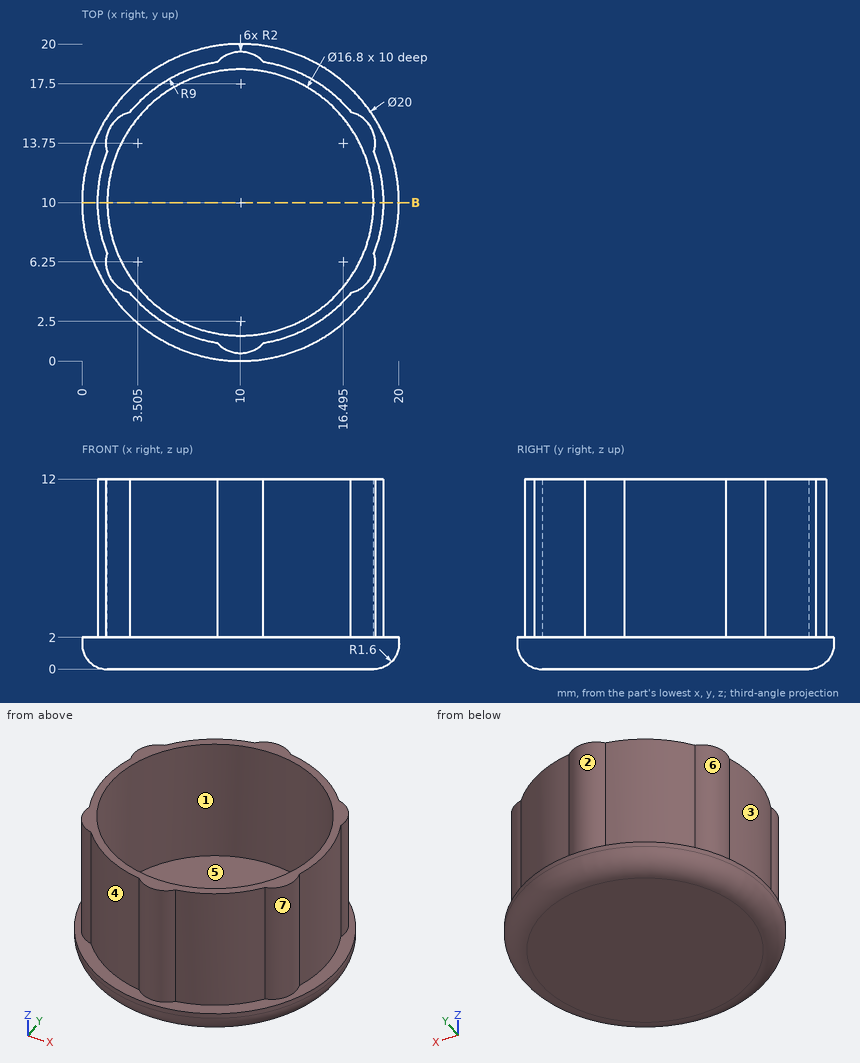
Drawing for the job (mm, zero at the part's lowest x, y, z). A direction names the side the tool comes from. Round coordinates to 2 decimals unless told otherwise and drop trailing zeros. Write each loop counter-clockwise with the first axis right and the second up, starting at its lowest first coordinate (ties: lowest second). Pieces come first, ordered by that corner, then holes. Notation, with made-up numbers: M 88.25,-13 L 103.25,-13 A11 cw 103.25,-2 Z; hole C 11,23.25 d9. An arc over 180 degrees is marked long. Answer in a Markdown table with one row per item.
1. Flat gauge pins, fed straight in: P1, Ø12, axis at x = 4.5, y = 15.5, coming from the -Z side; P2, Ø6, axis at x = 16, z = 10.5, coming from the +Y side (1 decimal); P3, Ø6, axis at x = 3, z = 2.5, coming from the +Y side; P4, Ø4, axis at x = 14, y = 10.5, coming from the +Z side. Where does each tip first touch, or does it go through?
Geometry check:
| item | result |
|---|---|
| P1 | z = 0 |
| P2 | y = 18.5 |
| P3 | y = 19.15 |
| P4 | z = 2 |
2. Saw through at B-B (y = 10). List the corners of the cut face in (x, z), and give its area (3 significant figures).
Geometry check:
| item | result |
|---|---|
| outline | M 0,1.6 A1.6 ccw 1.6,0 L 18.4,0 A1.6 ccw 20,1.6 L 20,2 L 19,2 L 19,12 L 18.4,12 L 18.4,2 L 1.6,2 L 1.6,12 L 1,12 L 1,2 L 0,2 Z |
| area | 50.9 mm2 |
3. Mould opens along X. For the marked faces 1, 2 and 3 say: +X half, -X half, draft (parallel to the pull), parting line (faces both ways), or undercut.
Geometry check:
| item | result |
|---|---|
| face 1 | undercut |
| face 2 | parting line |
| face 3 | -X half |
4. Probe L1, parallel to Z at x = 10.25, y = 9; L2, parallel to X at y = 7.75, z = 10.25; L3, parallel to Y at x = 17.5, z = 9.5. List the from-to ranges inside material, lowest first. Write a range as [from, to].
Geometry check:
| item | result |
|---|---|
| L1 | [0, 2] |
| L2 | [1.29, 1.91], [18.09, 18.71] |
| L3 | [4.52, 6.22], [13.78, 15.48] |
5. Which spindle directions (+Z, -Z, +X, -X, +Y, -Y) get a long thin tool onto all of the face, cutting with end or side? Do the marked faces 4, 5, 6 and 7. Say none if no direction does.
Geometry check:
| item | result |
|---|---|
| face 4 | +Z, -X, -Y |
| face 5 | +Z |
| face 6 | +Z, -X |
| face 7 | +Z, +X |
